```python
from build123d import *

# Parameters (mm, degrees)
SCHIZZO1_R                    = 14.03
ESTRUSIONE_ESTRUSIONE1_DEPTH  = 3.6
SCHIZZO2_R                    = 7.98
ESTRUSIONE_ESTRUSIONE2_DEPTH  = 13.53
SCHIZZO3_R                    = 14.03
ESTRUSIONE_ESTRUSIONE3_DEPTH  = 3.6
SCHIZZO4_R                    = 7.995
ESTRUSIONE_ESTRUSIONE4_DEPTH  = 6.2
ESTRUSIONE_ESTRUSIONE5_START  = 1.95
SCHIZZO5_R                    = 7.995
ESTRUSIONE_ESTRUSIONE5_DEPTH  = 1.95
SCHIZZO6_R                    = 7.915
ESTRUSIONE_ESTRUSIONE6_DEPTH  = 11.25
RACCORDO1_R                   = 2.5
FORO_FILETTATO_M3X0_5_1_D     = 2.5
FORO_FILETTATO_M3X0_5_1_DEPTH = 6.1
FORO_FILETTATO_M3X0_5_1_TIP   = 0.751075774
SCHIZZO10_R                   = 3
TAGLIO_ESTRUSIONE1_DEPTH      = 45.767160955
FORO_FILETTATO_M3X0_5_2_D     = 2.5
FORO_FILETTATO_M3X0_5_2_DEPTH = 8.5
FORO_FILETTATO_M3X0_5_2_TIP   = 0.751075774


with BuildPart() as part:
    # Schizzo1 → Estrusione-Estrusione1 (new body)
    with BuildSketch(Plane(origin=(0, 0, 0), x_dir=(1, 0, 0), z_dir=(0, 1, 0))):
        with Locations(Location((0, 0, 0), (0, 0, 270))):
            Circle(SCHIZZO1_R)
    extrude(amount=ESTRUSIONE_ESTRUSIONE1_DEPTH)

    # Schizzo2 → Estrusione-Estrusione2 (add)
    with BuildSketch(Plane(origin=(0, 3.6, 0), x_dir=(1, 0, 0), z_dir=(0, 1, 0))):
        with Locations(Location((0, 0, 0), (0, 0, 270))):
            Circle(SCHIZZO2_R)
    extrude(amount=ESTRUSIONE_ESTRUSIONE2_DEPTH)

    # Schizzo3 → Estrusione-Estrusione3 (add)
    with BuildSketch(Plane(origin=(0, 17.13, 0), x_dir=(1, 0, 0), z_dir=(0, 1, 0))):
        with Locations(Location((0, 0, 0), (0, 0, 270))):
            Circle(SCHIZZO3_R)
    extrude(amount=ESTRUSIONE_ESTRUSIONE3_DEPTH)

    # Schizzo4 → Estrusione-Estrusione4 (add)
    with BuildSketch(Plane(origin=(0, 20.73, 0), x_dir=(1, 0, 0), z_dir=(0, 1, 0))):
        with Locations(Location((0, 0, 0), (0, 0, 90))):
            Circle(SCHIZZO4_R)
    extrude(amount=ESTRUSIONE_ESTRUSIONE4_DEPTH)

    # Schizzo5 → Estrusione-Estrusione5 (add)
    with BuildSketch(Plane.XZ.offset(ESTRUSIONE_ESTRUSIONE5_START)):
        with Locations(Location((0, 0, 0), (0, 0, 270))):
            Circle(SCHIZZO5_R)
    extrude(amount=-ESTRUSIONE_ESTRUSIONE5_DEPTH)

    # Schizzo6 → Estrusione-Estrusione6 (add)
    with BuildSketch(Plane(origin=(0, 26.93, 0), x_dir=(1, 0, 0), z_dir=(0, 1, 0))):
        with Locations(Location((0, 0, 0), (0, 0, 90))):
            Circle(SCHIZZO6_R)
    extrude(amount=ESTRUSIONE_ESTRUSIONE6_DEPTH)

    # Raccordo1
    raccordo1_edges = [part.edges().sort_by_distance(p)[0] for p in [
        (0, 3.6, -7.98),
        (0, 17.13, -7.98),
    ]]
    fillet(raccordo1_edges, radius=RACCORDO1_R)

    # Foro filettato M3x0.5-1
    with Locations(Plane(origin=(0, 20.73, 0), x_dir=(1, 0, 0), z_dir=(0, 1, 0))):
        with Locations((0, 10.65), (10.65, 0), (-10.65, 0), (0, -10.65)):
            Hole(FORO_FILETTATO_M3X0_5_1_D / 2, depth=FORO_FILETTATO_M3X0_5_1_DEPTH)
            with Locations((0, 0, -(FORO_FILETTATO_M3X0_5_1_DEPTH + FORO_FILETTATO_M3X0_5_1_TIP / 2))):  # 118° drill point
                Cone(0, FORO_FILETTATO_M3X0_5_1_D / 2, FORO_FILETTATO_M3X0_5_1_TIP, mode=Mode.SUBTRACT)

    # Schizzo10 → Taglio-Estrusione1 (cut, through all)
    with BuildSketch(Plane(origin=(0, 38.18, 0), x_dir=(1, 0, 0), z_dir=(0, 1, 0))):
        with Locations(Location((0, 0, 0), (0, 0, 270))):
            Circle(SCHIZZO10_R)
    extrude(amount=-TAGLIO_ESTRUSIONE1_DEPTH, mode=Mode.SUBTRACT)

    # Foro filettato M3x0.5-2
    with Locations(Plane(origin=(0, 0, 0), x_dir=(-1, 0, 0), z_dir=(0, -1, 0))):
        with Locations((-10.030128499, 3.580366224), (-1.914376144, 10.476529195), (8.115752354, 6.896162971), (10.030128499, -3.580366224), (1.914376144, -10.476529195), (-8.115752354, -6.896162971), (0, 0)):
            Hole(FORO_FILETTATO_M3X0_5_2_D / 2, depth=FORO_FILETTATO_M3X0_5_2_DEPTH)
            with Locations((0, 0, -(FORO_FILETTATO_M3X0_5_2_DEPTH + FORO_FILETTATO_M3X0_5_2_TIP / 2))):  # 118° drill point
                Cone(0, FORO_FILETTATO_M3X0_5_2_D / 2, FORO_FILETTATO_M3X0_5_2_TIP, mode=Mode.SUBTRACT)


solid = part.part
```
Part model, mm, in its own coordinate system. A direction names the side the tool comes from. Give positions to 0.01 mm unless a question says otherwise; leave off trailing zeros. Loops run counter-clockwise (first coordinate to the right, second up) from the corner with the lowest first, then second, coordinate; pieces in that order, holes last. Notation, with made-up numbers: M 68.25,-13.75 L 82.25,-13.75 A28 ccw 82.25,5.25 Z; hole C 87,38 d1. An arc over 180 degrees is marked long. Return JSON: item names as keys, results as strings.
1) Saw through at D-D, the plane y = 1. List the corners of the cut face in (x, z).
Calculated:
{"outline": "C 0,0 d28.06; hole C -10.03,3.58 d2.5; hole C -8.12,-6.9 d2.5; hole C -1.91,10.48 d2.5; hole C 0,0 d6; hole C 1.91,-10.48 d2.5; hole C 8.12,6.9 d2.5; hole C 10.03,-3.58 d2.5"}
2) Drill centre lines: line 1 (Y direction, x = 5.5, z = -11.5); line 2 (Y direction, x = -1.75, z = -7.75); line 3 (Z direction, x = 7, y = 3). Where is each one in solid material? Low to high.
Calculated:
{"line 1": "y = 0 to 3.6, 17.13 to 20.73", "line 2": "y = -1.95 to 26.93", "line 3": "z = -12.16 to 6.33, 7.46 to 12.16"}
3) Saw through at A-A, the plane z = 0. Count the separate pieces of the cut face and the enclosed holes in it, then the cut area to 3 significant figures.
Calculated:
{"separate pieces": "4", "enclosed holes": "0", "area": "473 mm2"}
4) Pull direction Y, two halves, no side cores. Call faces 1 (the face through (-2, 17.13, -10.5)), 2 (the face through (-3.4, -1.95, 0.1)), 3 (the face through (4.214, 18.905, 13.382)): released by +Y, released by -Y, zero draft, split by the parting line, or undercut.
Calculated:
{"face 1": "undercut", "face 2": "released by -Y", "face 3": "zero draft"}
5) Saw through at B-B, the plane y = 29.5. List the corners of the cut face in (x, z) (3 decimals), then the cut area to 3 significant figures.
Calculated:
{"outline": "C 0,0 d15.83; hole C 0,0 d6", "area": "169 mm2"}
6) Flat gauge pins, fed straight in: pin 1 Ø2 at (y, z) = (23, -8) entering from +X; pin 2 Ø1.5 at (x, z) = (-4.5, -10) entering from -Y; pin 3 Ø1 at (y, z) = (18.5, -9.5) entering from +X. Where does each tip first touch, or does it go through?
Calculated:
{"pin 1": "stops at x = 3.86", "pin 2": "stops at y = 0", "pin 3": "stops at x = 10.76"}
7) 3-axis set-ups, long thin cutter, end or side, ignore diameter. For faces 4 (the face through (-9.4, 18.78, -0.05)), 5 (the face through (7.91, 10.31, -1.04)), 6 (the face through (4.214, 1.775, 13.382)), 7 (the face through (-2.077, 1.95, 9.237)): which of +Z, -Z, +X, -X, +Y, -Y reach the whole face in a straight line?
Calculated:
{"face 4": "+Y", "face 5": "none", "face 6": "+Y, -Y", "face 7": "-Y"}
